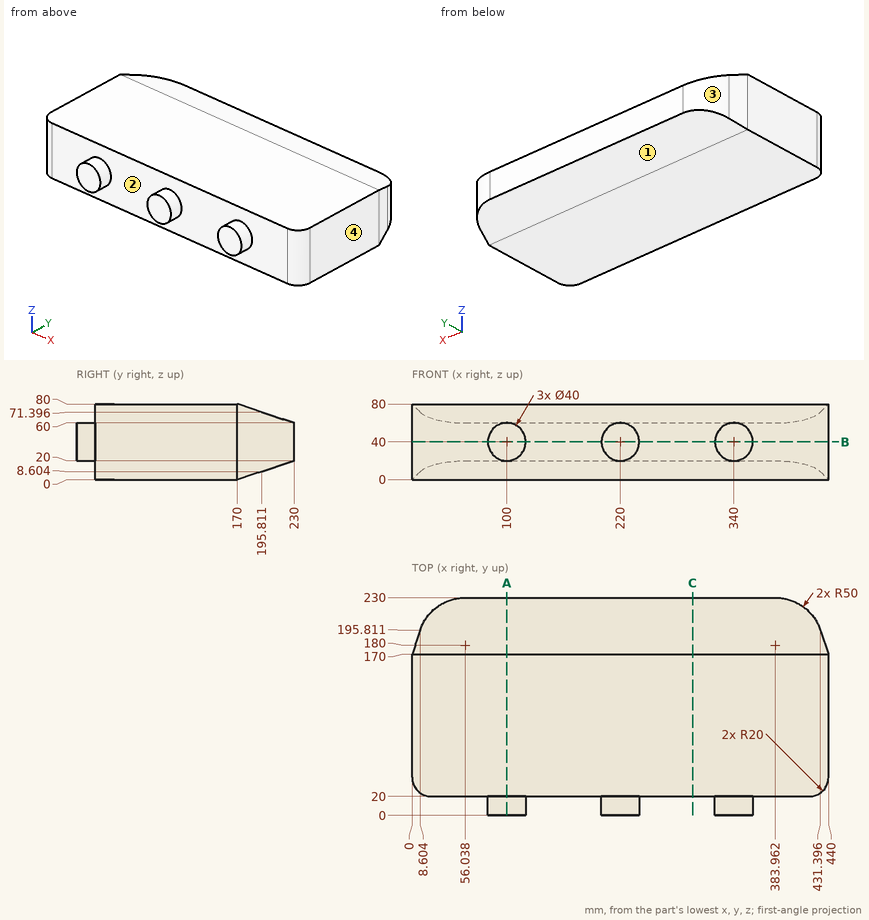
Input: dimensioned drawing with shaded views. Units: mm. Origin: part minimum x, y, z. Give positions to 0.01 mm unless a question says otherwise; leave off trailing zeros. Order: outer loops, then holes, each group sorted by start corner. A loop starts at its lowest first (then second) coordinate and runs counter-clockwise, first axis right, second up. Notation, with made-up numbers: (71.5, 17) -> (94.5, 17) arc R24 cw to (94.5, 43) -> close; hole circle Ø4 at (-10.5, 0.25). An arc over 180 degrees is marked (long way). Use a Markdown table: item, result.
1) Section query C-C, the plane x = 296.5. Return the cut outline in (y, z), then the cut area to 3 significant figures.
Answer list:
| item | result |
|---|---|
| outline | (20, 0) -> (170, 0) -> (230, 20) -> (230, 60) -> (170, 80) -> (20, 80) -> close |
| area | 15,600 mm² |
2) Section query A-A, the plane x = 100. Return the cut outline in (y, z), then the cut area to 3 significant figures.
Answer list:
| item | result |
|---|---|
| outline | (0, 20) -> (20, 20) -> (20, 0) -> (170, 0) -> (230, 20) -> (230, 60) -> (170, 80) -> (20, 80) -> (20, 60) -> (0, 60) -> close |
| area | 16,400 mm² |
3) Contact query for a flat-ended pin moving along its axis: P1, Ø2, axis at x = 99.5, y = 173.5, coming from the -Z side. Output: stop coordinate, or through.
Answer list:
| item | result |
|---|---|
| P1 | z = 0.83 |
4) Section query B-B, the plane z = 40. Return the cut outline in (x, y).
Answer list:
| item | result |
|---|---|
| outline | (0, 40) arc R20 ccw to (20, 20) -> (80, 20) -> (80, 0) -> (120, 0) -> (120, 20) -> (200, 20) -> (200, 0) -> (240, 0) -> (240, 20) -> (320, 20) -> (320, 0) -> (360, 0) -> (360, 20) -> (420, 20) arc R20 ccw to (440, 40) -> (440, 170) -> (431.4, 195.81) arc R50 ccw to (383.96, 230) -> (56.04, 230) arc R50 ccw to (8.6, 195.81) -> (0, 170) -> close |
5) Ray query, line 1 along Y through (x, z) = (317, 44); line 2 along X through (y, z) = (23.5, 31) (1 decimal); line 3 along Y through (x, z) = (411, 58). Return the intervals inside material, ascending. Write a range as [from, to].
Answer list:
| item | result |
|---|---|
| line 1 | [20, 230] |
| line 2 | [8.7, 431.3] |
| line 3 | [20, 222.06] |
6) Mould query, pull axis X, two halves, no side actions, for the marked faces 1, 2, 3 and 4. Classes: +X half, -X half, draft (parallel to the pull), parting line (faces both ways), or undercut.
Answer list:
| item | result |
|---|---|
| face 1 | draft |
| face 2 | undercut |
| face 3 | -X half |
| face 4 | +X half |
